Build history of the part. All positions in model axes, mm. A direction names the side the tool comes from. Round coordinates to 2 decimals unless told otherwise and drop trailing zeros. Loops run counter-clockwise (first coordinate to the right, second up) from the corner with the lowest first, then second, coordinate; pieces in that order, holes last. Notation, with made-up numbers: M 3.5,3 L 18.5,3 A20 cw 18.5,40 Z; hole C 23.25,7.5 d7. An arc over 180 degrees is marked long. One line per item, written item: value.
```python
from build123d import *

# Parameters (mm, degrees)
SKETCH_1_W     = 20
SKETCH_1_H     = 3
CHAMFER_1_SIZE = 0.5


# Read off the part's stored shape, not the designer's step: M3x0.5 ねじ穴2
with BuildPart() as part:
    # ｽｹｯﾁ1 → 回転1 (revolve)
    with BuildSketch(Plane.XY, mode=Mode.PRIVATE) as revolve_1_sk:
        with Locations((0, 1.5)):
            Rectangle(SKETCH_1_W, SKETCH_1_H)
    revolve(revolve_1_sk.sketch.rotate(Axis((0, 0, 0), (1, 0, 0)), 90), axis=Axis((0, 0, 0), (1, 0, 0)))

    # M3x0.5 ねじ穴2 outline → M3x0.5 ねじ穴2 (revolve, cut)
    with BuildSketch(Plane.YX):
        Polygon((0, 10), (0, 0.748924226), (1.25, 1.5), (1.25, 4), (1.5, 4), (1.5, 10), align=None)
        Polygon((1.25, -1.5), (0, -0.748924226), (0, -10), (1.5, -10), (1.5, -4), (1.25, -4), align=None)
    revolve(axis=Axis((0, 0, 0), (1, 0, 0)), mode=Mode.SUBTRACT)

    # 面取り1
    chamfer_1_edges = [part.edges().sort_by_distance(p)[0] for p in [
        (-10, 0, -3),
        (10, 0, -3),
    ]]
    chamfer(chamfer_1_edges, length=CHAMFER_1_SIZE)


solid = part.part
```
Item 1: Slice it at B-B, the plane x = 5. Give the cut face in (y, z), and give its area (3 significant figures).
Check values:
outline: C 0,0 d6; hole C 0,0 d3
area: 21.2 mm2
Item 2: Pull direction Z, two halves, no side cores. Call faces 1 (the face through (-10, 2, 0)), 2 (the face through (-0.87, -0.16, -0.12)), 3 (the face through (0.13, -0.9, 2.86)): pulls with the +Z half, pulls with the -Z half, needs draft (parallel to the pull), parting line crosses it, or undercut.
Check values:
face 1: needs draft
face 2: undercut
face 3: parting line crosses it
Item 3: Slice it at A-A, the plane x = -2. Give the cut face in (y, z).
Check values:
outline: C 0,0 d6; hole C 0,0 d2.5
Item 4: Which spindle directions (+Z, -Z, +X, -X, +Y, -Y) get a long thin tool onto all of the face, cutting with end or side? Do faces 4 (the face through (10, 2, 0)), 5 (the face through (2.77, -0.27, -1.22)), 6 (the face through (-2.73, -0.27, -1.22)). Say none if no direction does.
Check values:
face 4: +Z, -Z, +X, +Y, -Y
face 5: +X
face 6: -X
Item 5: Wall check: line 1 along Y through (x, z) = (-3, -0.5); line 2 along Z through (x, y) = (2.25, -2.6); line 3 along Y through (x, z) = (6.5, -1.05). Give the ranges that are in metal, low to high.
Check values:
line 1: y = -2.96 to -1.15, 1.15 to 2.96
line 2: z = -1.5 to 1.5
line 3: y = -2.81 to -1.07, 1.07 to 2.81
Item 6: Drop flat-ended pins along their axis: P1, Ø2, axis at x = 6.5, z = -1.5, coming from the -Y side; P2, Ø1.8, axis at y = 0, z = 0, coming from the +X side; P3, Ø2, axis at y = 0, z = 0, coming from the -X side. Give the stop position or say it passes through.
Check values:
P1: stops at y = -2.96
P2: stops at x = 1.29
P3: stops at x = -1.35
